For this review, take the finished solid that the model builds, in its own axes (mm). A direction names the side the tool comes from. Round coordinates to 2 decimals unless told otherwise and drop trailing zeros. Order: outer loops, then holes, each group sorted by start corner. A loop starts at its lowest first (then second) coordinate and runs counter-clockwise, first axis right, second up. Notation, with made-up numbers: (-0.5, 23) -> (36.5, 23) arc R22 ccw to (36.5, 52) -> close; hole circle Ø4 at (-34, -38.5). An arc over 180 degrees is marked (long way). Use a Markdown table: item, result. Add a question column.
1) Consider section A-A (x = -43). State the section outline as (y, z) points, plus the area to 3 significant figures.
2) Machinability: for faces 5 (the face through (-1, 2, 35)), 6 (the face through (-35, 2, 0)), which of the approach directions +Z, -Z, +X, -X, +Y, -Y give a long, thin tool a straight path to every point of the face, cutting with its end or side? Answer none if there is none.
3) Draft analysis for pull direction Z (two halves, no side actions). For faces 1 (the face through (36.6, 2.5, -31.2)), 2 (the face through (-1, 2, -35)), 3 (the face through (-53, 2, 0)), 4 (the face through (46, 2, -30)), state which applies: pulls with the +Z half, pulls with the -Z half, needs draft (parallel to the pull), parting line crosses it, or undercut.
4) Consider section C-C (z = 1.5). State the section outline as (x, y) points, plus the area to 3 significant figures.
5) Consider section B-B (x = 27.5). State the section outline as (y, z) points.
6) Wall thickness on line 1 along Z through (x, y) = (-37, 1.45); line 2 along Z through (x, y) = (-44, 1.85); line 3 along Z through (x, y) = (48, 1.2): over which ranges is each line inside the solid? List them lowest first. Write a range as [from, to].
7) Consider section D-D (y = 4.05). Give the number of separate pieces and of enclosed holes in the cut face, plus the area to 3 significant figures.
```python
from build123d import *

# Parameters (mm, degrees)
SKETCH1_W               = 120
SKETCH1_H               = 70
BOSS_EXTRUDE1_DEPTH     = 5
CUT_EXTRUDE1_DEPTH      = 70.641941386
CUT_EXTRUDE1_DEPTH_BACK = 70.641941386
SKETCH2_W               = 10
SKETCH2_H               = 14
CUT_EXTRUDE2_DEPTH      = 70.641941386
CUT_EXTRUDE2_DEPTH_BACK = 70.641941386
SKETCH3_W               = 7
SKETCH3_H               = 70
CUT_EXTRUDE3_DEPTH      = 64.710281745
CUT_EXTRUDE3_DEPTH_BACK = 64.710281745
SKETCH4_R               = 1.5


with BuildPart() as part:
    # Sketch1 → Boss-Extrude1 (new body)
    with BuildSketch(Plane(origin=(0, 0, 0), x_dir=(1, 0, 0), z_dir=(0, 1, 0))):
        Rectangle(SKETCH1_W, SKETCH1_H)
    extrude(amount=BOSS_EXTRUDE1_DEPTH)

    # Sketch2 → Cut-Extrude1 (cut, two sides: drawn at the far end of the back side and taken through both)
    with BuildSketch(Plane(origin=(0, 5, 0), x_dir=(1, 0, 0), z_dir=(0, 1, 0)).offset(-CUT_EXTRUDE1_DEPTH_BACK)):
        with Locations((-40, 0)):
            Rectangle(SKETCH2_W, SKETCH2_H)
    extrude(amount=CUT_EXTRUDE1_DEPTH + CUT_EXTRUDE1_DEPTH_BACK, mode=Mode.SUBTRACT)

    # Sketch3 → Cut-Extrude2 (cut, two sides: drawn at the far end of the back side and taken through both)
    with BuildSketch(Plane(origin=(0, 5, 0), x_dir=(1, 0, 0), z_dir=(0, 1, 0)).offset(-CUT_EXTRUDE2_DEPTH_BACK)):
        with Locations((56.5, 0)):
            Rectangle(SKETCH3_W, SKETCH3_H)
        with Locations((-56.5, 0)):
            Rectangle(SKETCH3_W, SKETCH3_H)
    extrude(amount=CUT_EXTRUDE2_DEPTH + CUT_EXTRUDE2_DEPTH_BACK, mode=Mode.SUBTRACT)

    # Sketch4 → Cut-Extrude3 (cut, two sides: drawn at the far end of the back side and taken through both)
    with BuildSketch(Plane(origin=(0, 5, 0), x_dir=(1, 0, 0), z_dir=(0, 1, 0)).offset(-CUT_EXTRUDE3_DEPTH_BACK)):
        with Locations(Location((-37.5, -30, 0), (0, 0, 270))):
            Circle(SKETCH4_R)
        with Locations(Location((-27.5, -30, 0), (0, 0, 270))):
            Circle(SKETCH4_R)
        with Locations(Location((-47.5, -30, 0), (0, 0, 270))):
            Circle(SKETCH4_R)
        with Locations(Location((27.5, -30, 0), (0, 0, 90))):
            Circle(SKETCH4_R)
        with Locations(Location((47.5, -30, 0), (0, 0, 90))):
            Circle(SKETCH4_R)
        with Locations(Location((37.5, -30, 0), (0, 0, 90))):
            Circle(SKETCH4_R)
        with Locations(Location((47.5, 30, 0), (0, 0, 270))):
            Circle(SKETCH4_R)
        with Locations(Location((37.5, 30, 0), (0, 0, 270))):
            Circle(SKETCH4_R)
        with Locations(Location((27.5, 30, 0), (0, 0, 270))):
            Circle(SKETCH4_R)
        with Locations(Location((-27.5, 30, 0), (0, 0, 90))):
            Circle(SKETCH4_R)
        with Locations(Location((-37.5, 30, 0), (0, 0, 90))):
            Circle(SKETCH4_R)
        with Locations(Location((-47.5, 30, 0), (0, 0, 90))):
            Circle(SKETCH4_R)
    extrude(amount=CUT_EXTRUDE3_DEPTH + CUT_EXTRUDE3_DEPTH_BACK, mode=Mode.SUBTRACT)


solid = part.part
```
Results list:
| question | item | result |
|---|---|---|
| 1 | outline | (0, -35) -> (5, -35) -> (5, -7) -> (0, -7) -> close; (0, 7) -> (5, 7) -> (5, 35) -> (0, 35) -> close |
| 1 | area | 280 mm2 |
| 2 | face 5 | +Z, +X, -X, +Y, -Y |
| 2 | face 6 | +Y, -Y |
| 3 | face 1 | undercut |
| 3 | face 2 | pulls with the -Z half |
| 3 | face 3 | needs draft |
| 3 | face 4 | undercut |
| 4 | outline | (-53, 0) -> (-45, 0) -> (-45, 5) -> (-53, 5) -> close; (-35, 0) -> (53, 0) -> (53, 5) -> (-35, 5) -> close |
| 4 | area | 480 mm2 |
| 5 | outline | (0, -35) -> (5, -35) -> (5, -31.5) -> (0, -31.5) -> close; (0, -28.5) -> (5, -28.5) -> (5, 28.5) -> (0, 28.5) -> close; (0, 31.5) -> (5, 31.5) -> (5, 35) -> (0, 35) -> close |
| 6 | line 1 | [-35, -31.41], [-28.59, -7], [7, 28.59], [31.41, 35] |
| 6 | line 2 | [-35, -7], [7, 35] |
| 6 | line 3 | [-35, -31.41], [-28.59, 28.59], [31.41, 35] |
| 7 | separate pieces | 1 |
| 7 | enclosed holes | 13 |
| 7 | area | 7,200 mm2 |
